Verification items for the finished model (mm, model axes). A direction names the side the tool comes from. Round coordinates to 2 decimals unless told otherwise and drop trailing zeros. Order: outer loops, then holes, each group sorted by start corner. A loop starts at its lowest first (then second) coordinate and runs counter-clockwise, first axis right, second up. Notation, with made-up numbers: (11, -6.5) -> (29, -6.5) arc R33 cw to (29, 32.5) -> close; hole circle Ø5 at (-30.5, 33). An arc over 180 degrees is marked (long way). Answer in a Markdown table with one row per item. Add a question column.
```python
from build123d import *

# Parameters (mm, degrees)
F0_W     = 38.1
F0_H     = 57.15
F1_DEPTH = 13.97
F2_R     = 15.875
F3_DEPTH = 25.4
F4_W     = 38.1
F4_H     = 6.731
F5_DEPTH = 7.62


with BuildPart() as f1:
    # F0 (on Top) → F1 (new body)
    with BuildSketch(Plane.XY):
        Rectangle(F0_W, F0_H)
    extrude(amount=F1_DEPTH)

    # F2 (on face) → F3 (cut)
    with BuildSketch(Plane.XY.offset(13.97)):
        Circle(F2_R)
    extrude(amount=-F3_DEPTH, mode=Mode.SUBTRACT)

    # F4 (on face) → F5 (join)
    with BuildSketch(Plane(origin=(0, 0, 0), x_dir=(1, 0, 0), z_dir=(0, 0, -1))):
        with Locations((0, 25.2095)):
            Rectangle(F4_W, F4_H)
        with Locations((0, -25.2095)):
            Rectangle(F4_W, F4_H)
    extrude(amount=F5_DEPTH)


solid = f1.part
```
1) Cross-section at C-C, the plane z = -1. Record the boundary of the cut face in (x, y) (3 decimals).
2) Thickness scan on L1, parallel to Y at x = 0, z = 4 (3 decimals); L2, parallel to Y at x = 17, z = -3.5 (3 decimals); L3, parallel to X at y = 4, z = 2.75. Record the ranges inside material, lowest first. Write a range as [from, to].
3) Depth check by flat-ended pin: P1, Ø1, axis at x = 1, y = 21, coming from the -Z side. Enter the tip coordinate at first touch or a pass-through.
4) Draft check along X on faces 3 (the face through (-19.05, 0, 6)), 4 (the face through (17, 0, 13.97)), 5 (the face through (-3.441, -15.497, 7.083)), 6 (the face through (19.05, 0, 6)). Enter one of: +X half, -X half, draft (parallel to the pull), parting line (faces both ways), or undercut.
5) Cross-section at B-B, the plane x = 0. Record the boundary of the cut face in (y, z) (3 decimals).
6) Cross-section at D-D, the plane z = 9.25. Record the boundary of the cut face in (x, y) (3 decimals).
7) Cross-section at A-A, the plane y = 0. Record the boundary of the cut face in (x, z) (3 decimals).
8) Tool access check on faces 1 (the face through (0, -21.844, -4)), 2 (the face through (0, -28.575, 3)). Record the directions out of +Z, -Z, +X, -X, +Y, -Y that give a thin tool (end or side, any length) a straight path to the whole face; none if there is none.
Results below:
| question | item | result |
|---|---|---|
| 1 | outline | (-19.05, -28.575) -> (19.05, -28.575) -> (19.05, -21.844) -> (-19.05, -21.844) -> close; (-19.05, 21.844) -> (19.05, 21.844) -> (19.05, 28.575) -> (-19.05, 28.575) -> close |
| 2 | L1 | [-28.575, -15.875], [15.875, 28.575] |
| 2 | L2 | [-28.575, -21.844], [21.844, 28.575] |
| 2 | L3 | [-19.05, -15.36], [15.36, 19.05] |
| 3 | P1 | z = 0 |
| 4 | face 3 | -X half |
| 4 | face 4 | draft |
| 4 | face 5 | undercut |
| 4 | face 6 | +X half |
| 5 | outline | (-28.575, -7.62) -> (-21.844, -7.62) -> (-21.844, 0) -> (-15.875, 0) -> (-15.875, 13.97) -> (-28.575, 13.97) -> close; (15.875, 0) -> (21.844, 0) -> (21.844, -7.62) -> (28.575, -7.62) -> (28.575, 13.97) -> (15.875, 13.97) -> close |
| 6 | outline | (-19.05, -28.575) -> (19.05, -28.575) -> (19.05, 28.575) -> (-19.05, 28.575) -> close; hole circle Ø31.75 at (0, 0) |
| 7 | outline | (-19.05, 0) -> (-15.875, 0) -> (-15.875, 13.97) -> (-19.05, 13.97) -> close; (15.875, 0) -> (19.05, 0) -> (19.05, 13.97) -> (15.875, 13.97) -> close |
| 8 | face 1 | -Z, +X, -X |
| 8 | face 2 | +Z, -Z, +X, -X, -Y |
